from build123d import *

# Parameters (mm, degrees)
EXTRUDE_1_DEPTH           = 10
HOLE_WIZARD_3_0_3_1_D     = 3
HOLE_WIZARD_3_0_3_1_DEPTH = 8.5
HOLE_WIZARD_3_0_3_1_TIP   = 0.901290929
EXTRUDE_START             = 6
SKETCH_4_R                = 1.5
EXTRUDE_2_DEPTH           = 6
CHAMFER_1_SIZE            = 0.5


with BuildPart() as part:
    # Эскиз1 → Бобышка-Вытянуть1 (new body)
    with BuildSketch(Plane(origin=(0, 0, 0), x_dir=(1, 0, 0), z_dir=(0, 1, 0))):
        Polygon((1.443375673, -2.5), (2.886751346, 0), (1.443375673, 2.5), (-1.443375673, 2.5), (-2.886751346, 0), (-1.443375673, -2.5), align=None)
    extrude(amount=EXTRUDE_1_DEPTH)

    # Диаметр отверстия Ø3.0 (3)1
    with Locations(Plane(origin=(0, 0, 0), x_dir=(-1, 0, 0), z_dir=(0, -1, 0))):
        with Locations((0, 0)):
            Hole(HOLE_WIZARD_3_0_3_1_D / 2, depth=HOLE_WIZARD_3_0_3_1_DEPTH)
            with Locations((0, 0, -(HOLE_WIZARD_3_0_3_1_DEPTH + HOLE_WIZARD_3_0_3_1_TIP / 2))):  # 118° drill point
                Cone(0, HOLE_WIZARD_3_0_3_1_D / 2, HOLE_WIZARD_3_0_3_1_TIP, mode=Mode.SUBTRACT)

    # Эскиз4 → Бобышка-Вытянуть2 (add)
    with BuildSketch(Plane(origin=(0, 10, 0), x_dir=(1, 0, 0), z_dir=(0, 1, 0)).offset(EXTRUDE_START)):
        with Locations(Location((0, 0, 0), (0, 0, 90))):
            Circle(SKETCH_4_R)
    extrude(amount=-EXTRUDE_2_DEPTH)

    # Фаска1
    chamfer_1_edges = [part.edges().sort_by_distance(p)[0] for p in [
        (-1.5, 0, 0),
        (0, 16, 1.5),
    ]]
    chamfer(chamfer_1_edges, length=CHAMFER_1_SIZE)


solid = part.part
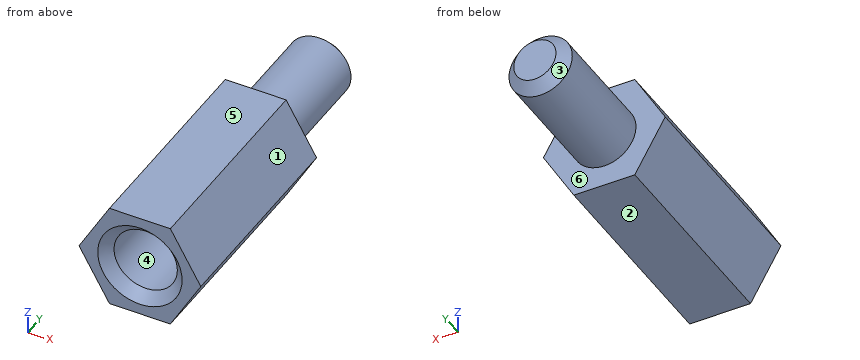
Input: part model. Units: mm. Frame: model coordinates. Face numbers are marked on the shaded views. A direction names the side the tool comes from. Coordinates: 2 decimals unless noted, no trailing zeros. Loops run counter-clockwise (first coordinate to the right, second up) from the corner with the lowest first, then second, coordinate; pieces in that order, holes last.
Q1. Material intervals for line 1 (Z direction, x = 0, y = 3); line 2 (Y direction, x = 0.15, z = 2.3); line 3 (X direction, y = 1, z = -0.75), sorted ascending.
Q2. Draft query along X for the marked faces 1, 2, 3 and 4. Return one class per face: +X half, -X half, draft (parallel to the pull), parting line (faces both ways), or undercut.
Q3. Cut plane B-B (x = 2.35). Output: boundary loops of the cut face in (y, z), then the cut area to 3 significant figures.
Q4. Cut plane A-A (y = 7.25). Output: boundary loops of the cut face in (x, z).
Q5. Contact query for flat-ended pins moving along their axis: pin 1 (2 mm diameter, centred on x = -1.5, z = -1, fed in from +Y); pin 2 (2 mm diameter, centred on x = -1, y = 12, fed in from -Z); pin 3 (1.5 mm diameter, centred on x = 1, y = 11.5, fed in from +Z); pin 4 (3 mm diameter, centred on y = 9.5, z = 2, fed in from -X). Output: stop coordinate, or through.
Q6. Set-up query: the marked faces 5 and 6. Return all of +Z, -Z, +X, -X, +Y, -Y with unobstructed straight access to the full face (end or side cutting, diameter ignored); none if empty.
Working result:
1. line 1: z = -2.5 to -1.5, 1.5 to 2.5
1. line 2: y = 0 to 10
1. line 3: x = -2.45 to -1.3, 1.3 to 2.45
2. face 1: +X half
2. face 2: draft
2. face 3: parting line
2. face 4: undercut
3. outline: (0, -0.93) - (10, -0.93) - (10, 0.93) - (0, 0.93) - close
3. area: 18.6 mm2
4. outline: (-2.89, 0) - (-1.44, -2.5) - (1.44, -2.5) - (2.89, 0) - (1.44, 2.5) - (-1.44, 2.5) - close; hole circle Ø3 at (0, 0)
5. pin 1: stops at y = 16
5. pin 2: stops at z = -1.5
5. pin 3: stops at z = 1.48
5. pin 4: stops at x = -2.6
6. face 5: +Z, +X, -X, +Y, -Y
6. face 6: +Y
